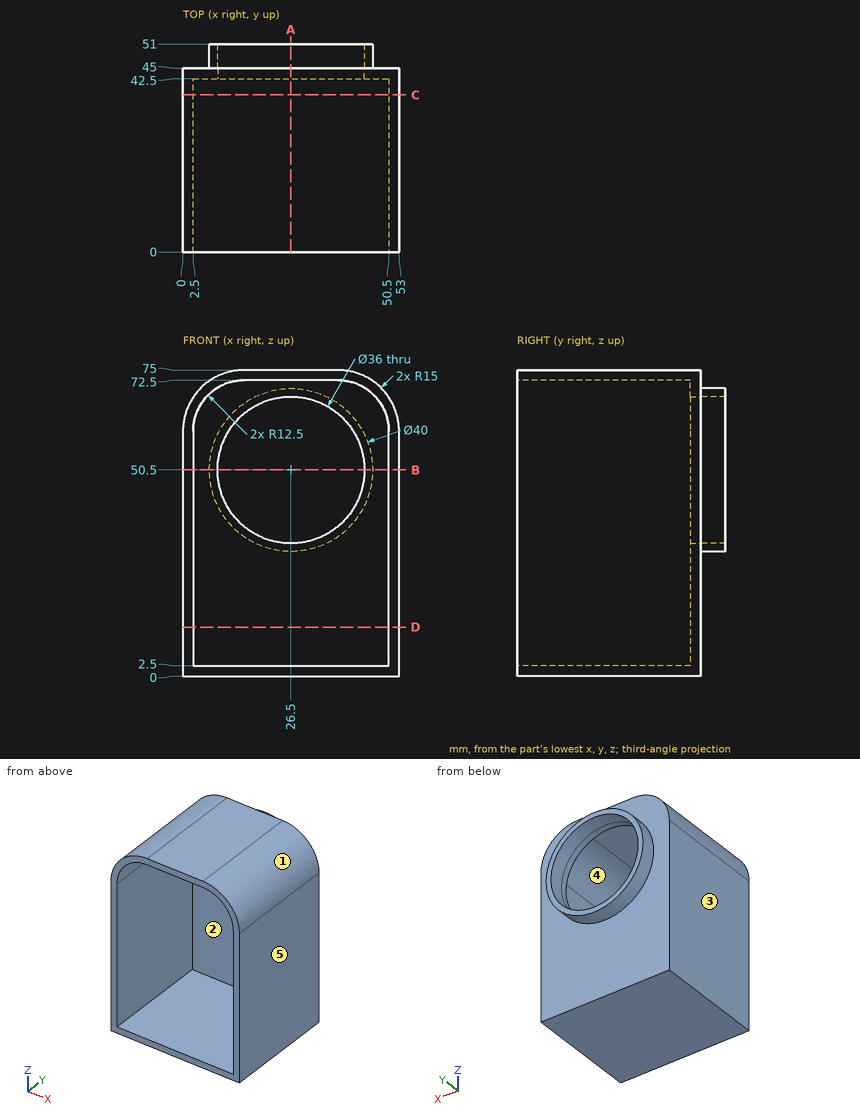
Here's the drawing with two shaded views (mm, measured from the low corner). I have some questions. A direction names the side the tool comes from. Give positions to 0.01 mm unless a question says otherwise; leave off trailing zeros. Loops run counter-clockwise (first coordinate to the right, second up) from the corner with the lowest first, then second, coordinate; pieces in that order, holes last. Notation, with made-up numbers: M 20,26.25 L 56,26.25 A16 cw 56,41.25 Z; hole C 44.5,10 d2. An arc over 180 degrees is marked long. One line per item, written item: value.
1) Imagine slicing it at A-A on x = 26.5. Write out the boundary of the cut face in (y, z).
Geometry check:
outline: M 0,0 L 45,0 L 45,30.5 L 51,30.5 L 51,32.5 L 42.5,32.5 L 42.5,2.5 L 0,2.5 Z; M 0,72.5 L 42.5,72.5 L 42.5,68.5 L 51,68.5 L 51,70.5 L 45,70.5 L 45,75 L 0,75 Z
2) I'm going to push a flat-ended pin straight in: pin 1 (24 mm diameter, centred on x = 21, z = 30, fed in from -Y). Where does the tip first touch, or does it pass through?
Geometry check:
pin 1: stops at y = 42.5
3) Please list where these lines run through material, in increasing order: line 1 (X direction, y = 2, z = 21); line 2 (X direction, y = 49, z = 50); line 3 (Z direction, x = 26.5, y = 43.9).
Geometry check:
line 1: x = 0 to 2.5, 50.5 to 53
line 2: x = 6.51 to 8.51, 44.49 to 46.49
line 3: z = 0 to 32.5, 68.5 to 75
4) Imagine slicing it at D-D on z = 12. Write out the boundary of the cut face in (x, y), and give its area (3 significant figures).
Geometry check:
outline: M 0,0 L 2.5,0 L 2.5,42.5 L 50.5,42.5 L 50.5,0 L 53,0 L 53,45 L 0,45 Z
area: 345 mm²
5) Imagine slicing it at B-B on z = 50.5. Write out the boundary of the cut face in (x, y), and give its area (3 significant figures).
Geometry check:
outline: M 0,0 L 2.5,0 L 2.5,42.5 L 8.5,42.5 L 8.5,51 L 6.5,51 L 6.5,45 L 0,45 Z; M 44.5,42.5 L 50.5,42.5 L 50.5,0 L 53,0 L 53,45 L 46.5,45 L 46.5,51 L 44.5,51 Z
area: 279 mm²
6) On a 3-axis mill with a long thin cutter (end or side, diameter ignored), from which of +Z, -Z, +X, -X, +Y, -Y can I reach the whole of each face in a straight line? I mean the marked faces 1 and 2. Say none if no direction works.
Geometry check:
face 1: +Z, +X, +Y, -Y
face 2: -Y
7) Imagine slicing it at C-C on y = 38.5. Write out the boundary of the cut face in (x, z), and give its area (3 significant figures).
Geometry check:
outline: M 0,0 L 53,0 L 53,60 A15 ccw 38,75 L 15,75 A15 ccw 0,60 Z; hole M 2.5,2.5 L 50.5,2.5 L 50.5,60 A12.5 ccw 38,72.5 L 15,72.5 A12.5 ccw 2.5,60 Z
area: 585 mm²
8) Thinking about a two-plate mould opening in X: for the marked faces 3, 4 and 5, which applies, +X half, -X half, draft (parallel to the pull), parting line (faces both ways), or undercut?
Geometry check:
face 3: -X half
face 4: undercut
face 5: +X half
